Read the model definition and answer for the solid it produces. Units are mm, in the model's axes. Face numbers are marked on the shaded views. A direction names the side the tool comes from. Coordinates: 2 decimals unless noted, no trailing zeros. Write each loop counter-clockwise with the first axis right and the second up, starting at its lowest first coordinate (ties: lowest second). Pieces come first, ordered by that corner, then holes.
1) Determine the mould class of the marked faces 3, 4 and 5 for opening direction X: +X half, -X half, draft (parallel to the pull), parting line (faces both ways), or undercut.
2) The part is cut by section B-B (y = 65). Determine the outline of the cut face in (x, z), then the cut area to 3 significant figures.
3) The part is cut by section C-C (x = 77). Determine the outline of the cut face in (y, z), then the cut area to 3 significant figures.
4) Find the intervals of material crossed by line 1 (Y direction, x = 64.2, z = 19.05); line 2 (X direction, y = -49.5, z = 11); line 3 (Z direction, x = 72.5, y = -109), in increasing order.
5) Which of the six approach directions +Z, -Z, +X, -X, +Y, -Y give full straight-line access (tool end or side, diameter ignored) to the marked faces 1 and 2?
6) The part is cut by section A-A (z = 10.25). Determine the outline of the cut face in (x, y).
7) This flat-tipped pin is pushed along its axis until it touches: pin 1 Ø4 at (x, y) = (69.74, -30.66) entering from +Z. Where does it stop, or does it pass through?
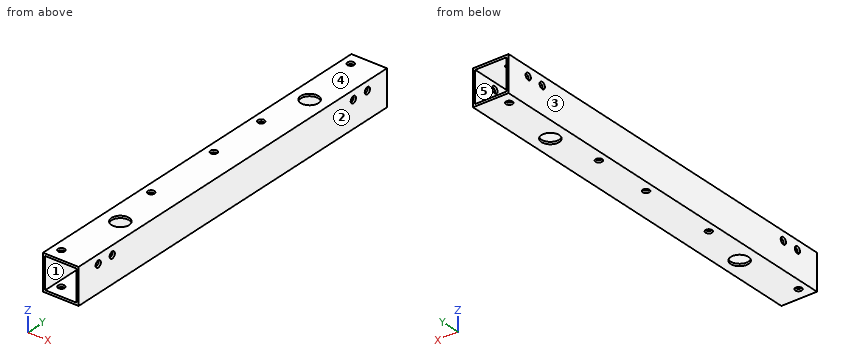
from build123d import *

# Parameters (mm, degrees)
SKETCH1_W                      = 25.4
SKETCH1_H                      = 279.4
BOSS_EXTRUDE1_DEPTH            = 25.4
SKETCH2_W                      = 22.225
SKETCH2_H                      = 22.225
CUT_EXTRUDE1_DEPTH             = 279.4
SKETCH3_R                      = 6.35
CUT_EXTRUDE2_DEPTH             = 25.4
F_3_16_0_1875_DIAMETER_HOLE2_D = 4.7625
F_3_16_0_1875_DIAMETER_HOLE3_D = 4.7625


with BuildPart() as part:
    # Sketch1 → Boss-Extrude1 (new body)
    with BuildSketch(Plane.XY):
        with Locations((76.086049872, -37.64964539)):
            Rectangle(SKETCH1_W, SKETCH1_H)
    extrude(amount=BOSS_EXTRUDE1_DEPTH)

    # Sketch2 → Cut-Extrude1 (cut)
    with BuildSketch(Plane(origin=(0, 102.05035461, 0), x_dir=(1, 0, 0), z_dir=(0, 1, 0))):
        with Locations((76.086049872, -12.7)):
            Rectangle(SKETCH2_W, SKETCH2_H)
    extrude(amount=-CUT_EXTRUDE1_DEPTH, mode=Mode.SUBTRACT)

    # Sketch3 → Cut-Extrude2 (cut)
    with BuildSketch(Plane(origin=(0, 0, 0), x_dir=(-1, 0, 0), z_dir=(0, 0, -1))):
        with Locations((-76.086049872, 48.07535461)):
            Circle(SKETCH3_R)
        with Locations((-76.086049872, -123.37464539)):
            Circle(SKETCH3_R)
    extrude(amount=-CUT_EXTRUDE2_DEPTH, mode=Mode.SUBTRACT)

    # 3/16 (0.1875) Diameter Hole2 (through all)
    with Locations(Plane(origin=(0, 0, 0), x_dir=(-1, 0, 0), z_dir=(0, 0, -1))):
        with Locations((-69.736049872, 93.41435461), (-69.736049872, 12.26135461), (-69.736049872, -30.66464539), (-69.736049872, -87.43364539), (-69.736049872, -168.71364539)):
            Hole(F_3_16_0_1875_DIAMETER_HOLE2_D / 2)

    # 3/16 (0.1875) Diameter Hole3 (through all)
    with Locations(Plane(origin=(88.786049872, 0, 0), x_dir=(0, 0, -1), z_dir=(1, 0, 0))):
        with Locations((-19.05, -159.56964539), (-19.05, -146.86964539), (-19.05, 71.57035461), (-19.05, 84.27035461)):
            Hole(F_3_16_0_1875_DIAMETER_HOLE3_D / 2)


solid = part.part
Reported:
1. face 3: -X half
1. face 4: draft
1. face 5: undercut
2. outline: (63.39, 0) - (88.79, 0) - (88.79, 25.4) - (63.39, 25.4) - close; hole (64.97, 1.59) - (87.2, 1.59) - (87.2, 23.81) - (64.97, 23.81) - close
2. area: 151 mm2
3. outline: (-177.35, 0) - (-129.66, 0) - (-129.66, 1.59) - (-177.35, 1.59) - close; (-177.35, 23.81) - (-129.66, 23.81) - (-129.66, 25.4) - (-177.35, 25.4) - close; (-117.09, 0) - (41.79, 0) - (41.79, 1.59) - (-117.09, 1.59) - close; (-117.09, 23.81) - (41.79, 23.81) - (41.79, 25.4) - (-117.09, 25.4) - close; (54.36, 0) - (102.05, 0) - (102.05, 1.59) - (54.36, 1.59) - close; (54.36, 23.81) - (102.05, 23.81) - (102.05, 25.4) - (54.36, 25.4) - close
3. area: 807 mm2
4. line 1: y = -177.35 to -161.95, -157.19 to -149.25, -144.49 to 69.19, 73.95 to 81.89, 86.65 to 102.05
4. line 2: x = 63.39 to 64.97, 87.2 to 88.79
4. line 3: z = 0 to 1.59, 23.81 to 25.4
5. face 1: +Y, -Y
5. face 2: +Z, -Z, +X, +Y, -Y
6. outline: (63.39, -177.35) - (64.97, -177.35) - (64.97, 102.05) - (63.39, 102.05) - close; (87.2, -177.35) - (88.79, -177.35) - (88.79, 102.05) - (87.2, 102.05) - close
7. pin 1: passes through
